```python
from build123d import *

# Parameters (mm, degrees)
SKETCH1_R           = 100
SKETCH1_R_2         = 25
BOSS_EXTRUDE1_DEPTH = 14.5
CUT_EXTRUDE1_DEPTH  = 12.5


with BuildPart() as part:
    # Sketch1 → Boss-Extrude1 (new, symmetric)
    with BuildSketch(Plane.XY):
        with Locations(Location((0, 0, 0), (0, 0, 180))):
            Circle(SKETCH1_R)
        with Locations(Location((0, 0, 0), (0, 0, 180))):
            Circle(SKETCH1_R_2, mode=Mode.SUBTRACT)
    extrude(amount=BOSS_EXTRUDE1_DEPTH, both=True)

    # Sketch2 → Cut-Extrude1 (cut, symmetric)
    with BuildSketch(Plane.XY):
        Polygon((100, 5), (110, -5), (100, -5), (60, -5), (60, 5), align=None)
        Polygon((57.346189113, -18.341608279), (94.301370413, -33.648945574), (99.713331414, -46.714575223), (90.474536089, -42.887740899), (53.519354789, -27.580403604), align=None)
        Polygon((45.961940777, -38.890872965), (74.246212025, -67.175144213), (74.246212025, -81.317279836), (67.175144213, -74.246212025), (38.890872965, -45.961940777), align=None)
        Polygon((27.580403604, -53.519354789), (42.887740899, -90.474536089), (37.475779898, -103.540165738), (33.648945574, -94.301370413), (18.341608279, -57.346189113), align=None)
        Polygon((5, -60), (5, -100), (-5, -110), (-5, -100), (-5, -60), align=None)
        Polygon((-18.341608279, -57.346189113), (-33.648945574, -94.301370413), (-46.714575223, -99.713331414), (-42.887740899, -90.474536089), (-27.580403604, -53.519354789), align=None)
        Polygon((-38.890872965, -45.961940777), (-67.175144213, -74.246212025), (-81.317279836, -74.246212025), (-74.246212025, -67.175144213), (-45.961940777, -38.890872965), align=None)
        Polygon((-53.519354789, -27.580403604), (-90.474536089, -42.887740899), (-103.540165738, -37.475779898), (-94.301370413, -33.648945574), (-57.346189113, -18.341608279), align=None)
        Polygon((-60, -5), (-100, -5), (-110, 5), (-100, 5), (-60, 5), align=None)
        Polygon((-57.346189113, 18.341608279), (-94.301370413, 33.648945574), (-99.713331414, 46.714575223), (-90.474536089, 42.887740899), (-53.519354789, 27.580403604), align=None)
        Polygon((-45.961940777, 38.890872965), (-74.246212025, 67.175144213), (-74.246212025, 81.317279836), (-67.175144213, 74.246212025), (-38.890872965, 45.961940777), align=None)
        Polygon((-27.580403604, 53.519354789), (-42.887740899, 90.474536089), (-37.475779898, 103.540165738), (-33.648945574, 94.301370413), (-18.341608279, 57.346189113), align=None)
        Polygon((-5, 60), (-5, 100), (5, 110), (5, 100), (5, 60), align=None)
        Polygon((18.341608279, 57.346189113), (33.648945574, 94.301370413), (46.714575223, 99.713331414), (42.887740899, 90.474536089), (27.580403604, 53.519354789), align=None)
        Polygon((38.890872965, 45.961940777), (67.175144213, 74.246212025), (81.317279836, 74.246212025), (74.246212025, 67.175144213), (45.961940777, 38.890872965), align=None)
        Polygon((53.519354789, 27.580403604), (90.474536089, 42.887740899), (103.540165738, 37.475779898), (94.301370413, 33.648945574), (57.346189113, 18.341608279), align=None)
    extrude(amount=CUT_EXTRUDE1_DEPTH, both=True, mode=Mode.SUBTRACT)


solid = part.part
```
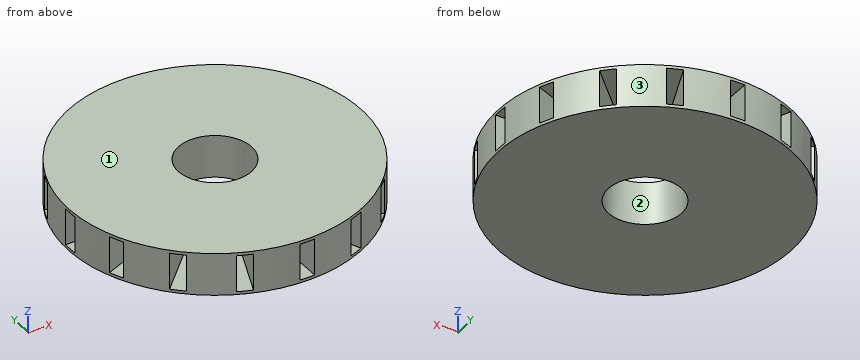
Read the model definition and answer for the solid it produces. Units are mm, in the model's axes. Face numbers are marked on the shaded views. Give positions to 0.01 mm unless a question says otherwise; leave off trailing zeros. Write each loop counter-clockwise with the first axis right and the second up, starting at its lowest first coordinate (ties: lowest second). Pieces come first, ordered by that corner, then holes. Notation, with made-up numbers: (54.5, 68) - (64.5, 68) arc R33 ccw to (64.5, 96) - close; hole circle Ø2 at (37.5, 23). An arc over 180 degrees is marked (long way). Write item = value, one per line. Start each with the question number.
Item 1: Each of these flat-tipped pins is pushed along its axis until it touches: P1, Ø1, axis at x = -26, z = 7, coming from the -Y side; P2, Ø4, axis at x = -68.5, z = 8, coming from the -Y side; P3, Ø8, axis at x = 1.5, z = 3.5, coming from the +Y side. Where does it stop, or does it pass through?
Item 2: Find section C-C (x = 79.5). Give the vertices of the cut face in (y, z), then the cut area to 3 significant figures.
Item 3: The mould has two halves that part along X. Classify the marked faces 1, 2 and 3: +X half, -X half, draft (parallel to the pull), parting line (faces both ways), or undercut.
Item 4: Find the intervals of material crossed by probe 1 along Y at (x, z) = (0, 4); probe 2 along X at (y, z) = (69.5, -6.25); probe 3 along X at (y, z) = (74, -6), in increasing order. Write a range as [from, to].
Item 5: Find section D-D (y = 84.5). Give the vertices of the cut face in (x, z), then the cut area to 3 significant figures.
Item 6: Find section A-A (y = 0). Give the vertices of the cut face in (x, z).
Response:
q1.P1 = -96.69
q1.P2 = -74.68
q1.P3 = 99.87
q2.outline = (-60.66, -14.5) - (60.66, -14.5) - (60.66, 14.5) - (-60.66, 14.5) - close; hole (-38.34, -12.5) - (-27.52, -12.5) - (-27.52, 12.5) - (-38.34, 12.5) - close; hole (-5, -12.5) - (5, -12.5) - (5, 12.5) - (-5, 12.5) - close; hole (27.52, -12.5) - (38.34, -12.5) - (38.34, 12.5) - (27.52, 12.5) - close
q2.area = 2,730 mm²
q3.face_1 = draft
q3.face_2 = undercut
q3.face_3 = parting line
q4.probe_1 = [-60, -25], [25, 60]
q4.probe_2 = [-62.43, -34.2], [-23.38, -5], [5, 23.38], [34.2, 62.43]
q4.probe_3 = [-66.93, -36.06], [-25.24, -5], [5, 25.24], [36.06, 66.93]
q5.outline = (-53.48, -14.5) - (53.48, -14.5) - (53.48, 14.5) - (-53.48, 14.5) - close; hole (-40.41, -12.5) - (-29.59, -12.5) - (-29.59, 12.5) - (-40.41, 12.5) - close; hole (-5, -12.5) - (5, -12.5) - (5, 12.5) - (-5, 12.5) - close; hole (29.59, -12.5) - (40.41, -12.5) - (40.41, 12.5) - (29.59, 12.5) - close
q5.area = 2,310 mm²
q6.outline = (-100, -14.5) - (-25, -14.5) - (-25, 14.5) - (-100, 14.5) - (-100, 12.5) - (-60, 12.5) - (-60, -12.5) - (-100, -12.5) - close; (25, -14.5) - (100, -14.5) - (100, -12.5) - (60, -12.5) - (60, 12.5) - (100, 12.5) - (100, 14.5) - (25, 14.5) - close
